The drawing under review shows one solid part. Ordinate dimensions are in mm from its lowest x, y, z. Round coordinates to 2 decimals unless told otherwise and drop trailing zeros. Write each loop counter-clockwise with the first axis right and the second up, starting at its lowest first coordinate (ties: lowest second). Pieces come first, ordered by that corner, then holes. Notation, with made-up numbers: M 45.25,50.5 L 49.25,50.5 A15 cw 49.25,73.5 Z; hole C 52,-6 d10. An arc over 180 degrees is marked long. One line per item, written item: value. Start each with the question number.
1) For P1, Ø2, axis at x = 74.5, z = 10, coming from the +Y side (1 decimal); P2, Ø6, axis at x = 128.5, z = 3, coming from the +Y side (1 decimal); P3, Ø5, axis at y = 59.5, z = 8, coming from the +X side (1 decimal), all flat-tipped, find the tip position at first contact; note any pin that passes through.
2) Take a section at D-D, the plane x = 141.5. Write out the cut boundary in (y, z), and give its area (3 significant figures).
3) Take a section at A-A, the plane y = 55.5. Write out the cut boundary in (x, z) (1 decimal).
4) Take a section at C-C, the plane x = 34.5. Write out the cut boundary in (y, z).
5) Wall thickness on probe 1 along X at (y, z) = (224, 10.25) (1 decimal); probe 2 along X at (y, z) = (206, 1) (1 decimal); probe 3 along Y at (x, z) = (35.5, 0.75) (1 decimal): over which ranges is each line inside the solid? List them lowest first.
6) Take a section at B-B, the plane z = 2. Write out the cut boundary in (x, y).
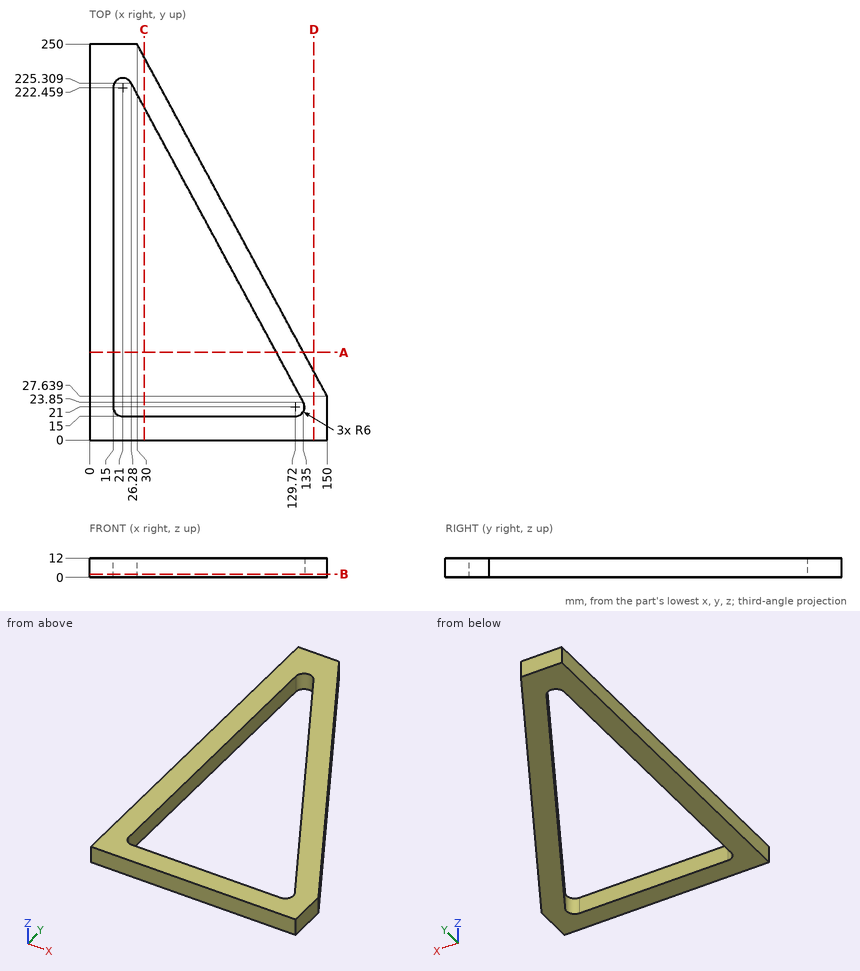
Checked values:
1. P1: stops at y = 169.4
1. P2: stops at y = 73
1. P3: stops at x = 134.2
2. outline: M 0,0 L 43.39,0 L 43.39,12 L 0,12 Z
2. area: 521 mm2
3. outline: M 0,0 L 15,0 L 15,12 L 0,12 Z; M 117.9,0 L 135,0 L 135,12 L 117.9,12 Z
4. outline: M 0,0 L 15,0 L 15,12 L 0,12 Z; M 210.08,0 L 241.66,0 L 241.66,12 L 210.08,12 Z
5. probe 1: x = 0 to 15.2, 27 to 44
5. probe 2: x = 0 to 15, 36.7 to 53.7
5. probe 3: y = 0 to 15, 208.2 to 239.8
6. outline: M 0,0 L 150,0 L 150,27.64 L 30,250 L 0,250 Z; hole M 15,21 A6 ccw 21,15 L 129.72,15 A6 ccw 135,23.85 L 26.28,225.31 A6 ccw 15,222.46 Z
